For this review, use the dimensioned drawing (mm, ordinates from the lowest corner) and the shaded views. A direction names the side the tool comes from. Coordinates: 2 decimals unless noted, no trailing zeros. Order: outer loops, then holes, each group sorted by start corner. A loop starts at its lowest first (then second) coordinate and runs counter-clockwise, first axis right, second up. Notation, with made-up numbers: M 23.25,82 L 56.25,82 A15 cw 56.25,107 Z; hole C -3.75,73 d5. An arc over 180 degrees is marked long. Write each question's results on one line, items separated by ' | '.
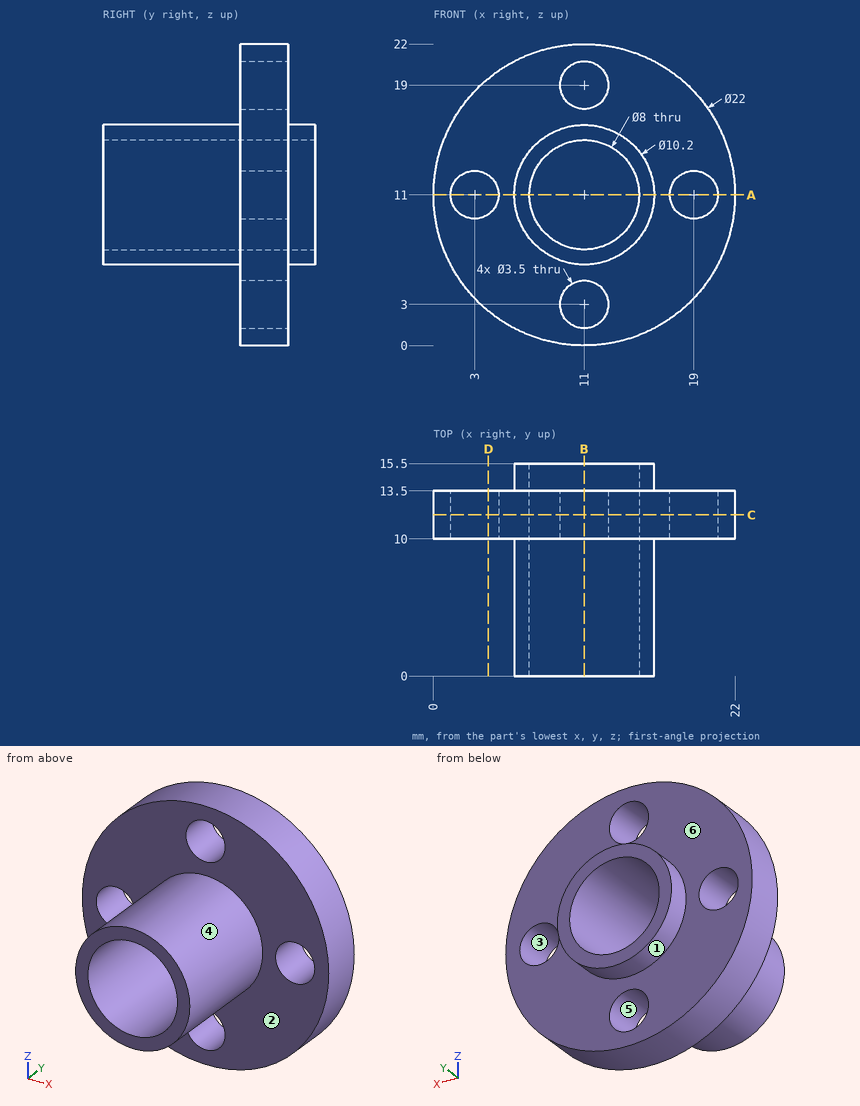
1) For pin 1 (1 mm diameter, centred on x = 18.5, z = 18, fed in from +Y); pin 2 (4 mm diameter, centred on x = 3, z = 11, fed in from -Y); pin 3 (4 mm diameter, centred on y = 5, z = 11, fed in from -X), all flat-tipped, find the tip position at first contact; note any pin that passes through.
Solutions:
pin 1: y = 13.5 | pin 2: y = 10 | pin 3: x = 5.9
2) Take a section at C-C on y = 11.75. State the section outline as (x, z) points, plus the area to 3 significant figures.
Solutions:
outline: C 11,11 d22; hole C 3,11 d3.5; hole C 11,11 d8; hole C 11,3 d3.5; hole C 11,19 d3.5; hole C 19,11 d3.5 | area: 291 mm2
3) The part is to be moulded in two halves that separate along Z. For the marked faces 1, 2 and 3, say which applies: pulls with the +Z half, pulls with the -Z half, needs draft (parallel to the pull), parting line crosses it, or undercut.
Solutions:
face 1: parting line crosses it | face 2: needs draft | face 3: undercut
4) Take a section at D-D on x = 4. State the section outline as (y, z) points, plus the area to 3 significant figures.
Solutions:
outline: M 10,2.51 L 13.5,2.51 L 13.5,9.56 L 10,9.56 Z; M 10,12.44 L 13.5,12.44 L 13.5,19.49 L 10,19.49 Z | area: 49.3 mm2
5) To check wall thickness, follow line 1 along X through (y, z) = (12.25, 11); line 2 along X through (y, z) = (4, 11). State the ranges of each line that lie inside material, in increasing order.
Solutions:
line 1: 0 to 1.25, 4.75 to 7, 15 to 17.25, 20.75 to 22 | line 2: 5.9 to 7, 15 to 16.1
6) Take a section at A-A on z = 11. State the section outline as (x, y) points.
Solutions:
outline: M 0,10 L 1.25,10 L 1.25,13.5 L 0,13.5 Z; M 4.75,10 L 5.9,10 L 5.9,0 L 7,0 L 7,15.5 L 5.9,15.5 L 5.9,13.5 L 4.75,13.5 Z; M 15,0 L 16.1,0 L 16.1,10 L 17.25,10 L 17.25,13.5 L 16.1,13.5 L 16.1,15.5 L 15,15.5 Z; M 20.75,10 L 22,10 L 22,13.5 L 20.75,13.5 Z
7) Take a section at B-B on x = 11. State the section outline as (y, z) points.
Solutions:
outline: M 0,5.9 L 10,5.9 L 10,4.75 L 13.5,4.75 L 13.5,5.9 L 15.5,5.9 L 15.5,7 L 0,7 Z; M 0,15 L 15.5,15 L 15.5,16.1 L 13.5,16.1 L 13.5,17.25 L 10,17.25 L 10,16.1 L 0,16.1 Z; M 10,0 L 13.5,0 L 13.5,1.25 L 10,1.25 Z; M 10,20.75 L 13.5,20.75 L 13.5,22 L 10,22 Z
8) For the marked faces 4, 5 and 6, list the 3-axis set-ups (+Z, -Z, +X, -X, +Y, -Y) from which the entire face can be reached by the end or side of a thin tool; tool diameter is ignored.
Solutions:
face 4: -Y | face 5: +Y, -Y | face 6: +Y
